from build123d import *

# Parameters (mm, degrees)
F0_R     = 25.4
F1_DEPTH = 6.35
F2_R     = 3.489483
F2_R_2   = 6.893113
F3_DEPTH = 6.35


with BuildPart() as f1:
    # F0 (on Front) → F1 (new body)
    with BuildSketch(Plane.XZ):
        Circle(F0_R)
    extrude(amount=F1_DEPTH)

    # F2 (on face) → F3 (cut)
    with BuildSketch(Plane.XZ.offset(6.35)):
        with Locations((-9.59337, 8.569406)):
            Circle(F2_R)
        with Locations((8.605205, 8.999294)):
            Circle(F2_R_2)
        with BuildLine():
            add(Edge.make_bspline(
                [(5.309401, -4.040631), (7.505178, -1.155375), (-1.556812, 3.462944), (-10.618802, 8.081263), (-3.752589, 0.577687), (3.113625, -6.925888), (5.309401, -4.040631)],
                knots=[0, 0, 0, 2.094395, 2.094395, 4.18879, 4.18879, 6.283185, 6.283185, 6.283185], degree=2, weights=[1, 0.5, 1, 0.5, 1, 0.5, 1]))
        make_face()
        with BuildLine():
            Line((13.33397, -12.351792), (-15.755093, -5.47359))
            ThreePointArc((-15.755093, -5.47359), (-3.738986, -19.605821), (13.33397, -12.351792))
        make_face()
    extrude(amount=-F3_DEPTH, mode=Mode.SUBTRACT)


solid = f1.part
Can you work these out from the model? Positions are in its coordinate system, mm. A direction names the side the tool comes from. Coordinates: 2 decimals unless noted, no trailing zeros. Write each loop counter-clockwise with the first axis right and the second up, starting at its lowest first coordinate (ties: lowest second). Pieces come first, ordered by that corner, then holes. Notation, with made-up numbers: (87, 70.25) -> (106, 70.25) arc R34 cw to (106, 107.25) -> close; hole circle Ø7 at (-32, 60.25). An arc over 180 degrees is marked (long way). Answer as CSV lines item,"result".
1) If we section it at C-C on z = -15: Please give me the cut outline in (x, y), then the cut area to 3 significant figures.
Check result:
outline,"(-20.5, -6.35) -> (-11.63, -6.35) -> (-11.63, 0) -> (-20.5, 0) -> close; (11.36, -6.35) -> (20.5, -6.35) -> (20.5, 0) -> (11.36, 0) -> close"
area,"114 mm²"
2) If we section it at D-D on x = 8.5: Please give me the cut outline in (y, z).
Check result:
outline,"(-6.35, -23.94) -> (0, -23.94) -> (0, -17.43) -> (-6.35, -17.43) -> close; (-6.35, -11.21) -> (0, -11.21) -> (0, 2.11) -> (-6.35, 2.11) -> close; (-6.35, 15.89) -> (0, 15.89) -> (0, 23.94) -> (-6.35, 23.94) -> close"
3) If we section it at B-B on z = -9: Please give me the cut outline in (x, y).
Check result:
outline,"(-23.75, -6.35) -> (-15.09, -6.35) -> (-15.09, 0) -> (-23.75, 0) -> close; (-0.84, -6.35) -> (23.75, -6.35) -> (23.75, 0) -> (-0.84, 0) -> close"
4) Will these pins go through, and if not, where does the flat tip stop? P1, Ø1, axis at y = -5.5, z = -19, coming from the -X side; P2, Ø8, axis at x = -9.59, z = 8.57, coming from the +Y side; P3, Ø1.5, axis at x = 14.5, y = -1, coming from the +Z side; P4, Ø6, axis at x = 8, z = 8, coming from the +Y side.
Check result:
P1,"x = -17.4"
P2,"y = 0"
P3,"z = 21.36"
P4,"through"
5) If I drill on line 1 (Z direction, x = 3.5, y = -1); line 2 (X direction, y = -5.5, z = 7.5); line 3 (Z direction, x = 4.5, y = -5.25), over which ranges is the centre line in solid material (lowest first)? Write a range as from..to.
Check result:
line 1,"-25.16..-19.6, -10.03..-4.24, -0.31..4.37, 13.63..25.16"
line 2,"-24.27..-12.91, -6.27..1.88, 15.33..24.27"
line 3,"-25..-19.32, -10.26..-4.37, -1.47..3.46, 14.54..25"
6) If we section it at A-A on x = -10: Please give me the cut outline in (y, z).
Check result:
outline,"(-6.35, -23.35) -> (0, -23.35) -> (0, -16.53) -> (-6.35, -16.53) -> close; (-6.35, -6.83) -> (0, -6.83) -> (0, 5.1) -> (-6.35, 5.1) -> close; (-6.35, 12.04) -> (0, 12.04) -> (0, 23.35) -> (-6.35, 23.35) -> close"
7) On a 3-axis mill with a long thin cutter (end or side, diameter ignored), from which of +Z, -Z, +X, -X, +Y, -Y can I reach the whole of each face in a straight line? I mean faces 1 (the flat face through (5, 0, 0)), 2 (the flat face through (-1.01, -3.22, -8.96)). Say none if no direction works.
Check result:
face 1,"+Z, -Z, +X, -X, +Y"
face 2,"+Y, -Y"
